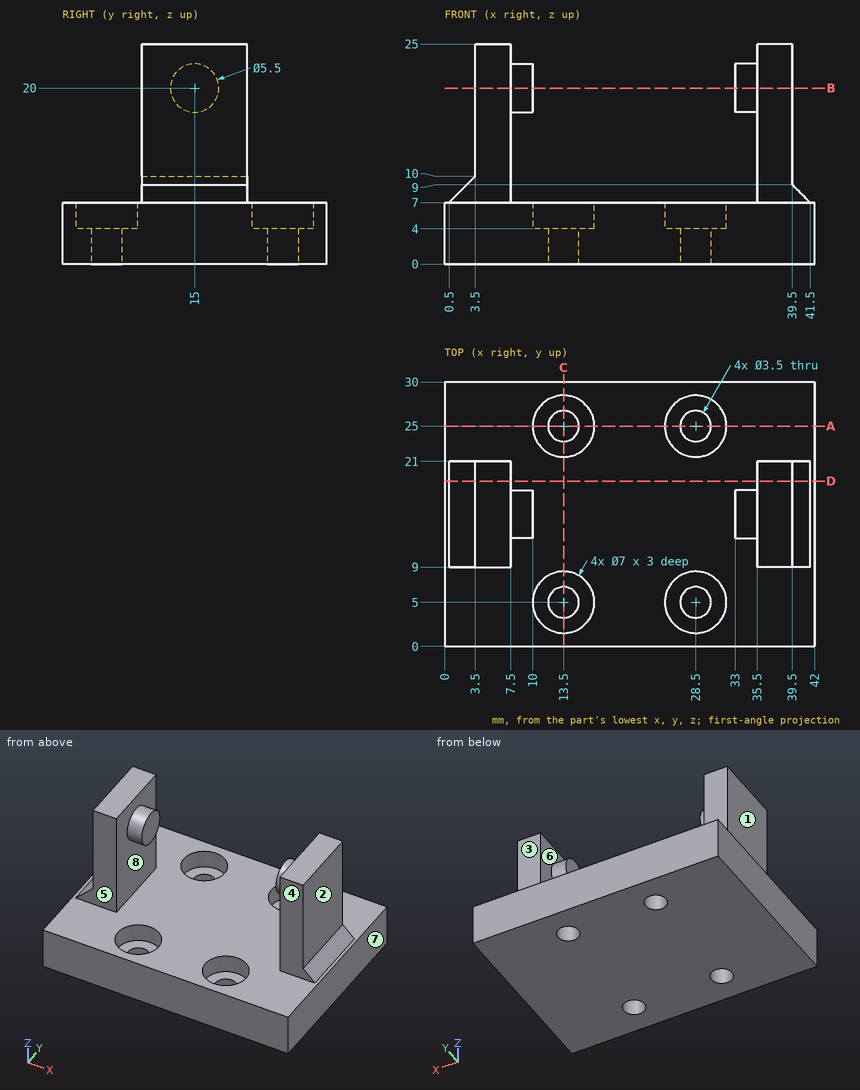
Design review of the part shown in the three views and the two pictorial views. Dimensions are in mm from the part's minimum x, y and z. A direction names the side the tool comes from. Round coordinates to 2 decimals unless told otherwise and drop trailing zeros. Write each loop counter-clockwise with the first axis right and the second up, starting at its lowest first coordinate (ties: lowest second). Pieces come first, ordered by that corner, then holes. Notation, with made-up numbers: M 73.25,42.5 L 118.25,42.5 A26 ccw 118.25,79.5 Z; hole C 33,46 d2. An arc over 180 degrees is marked long. One line per item, written item: value. Start each with the question number.
1. Take a section at B-B on z = 20. State the section outline as (x, y) points, then the cut area to 4 significant figures.
2. Take a section at D-D on y = 18.75. State the section outline as (x, z) points.
3. To check wall thickness, follow probe 1 along Y at (x, z) = (28.5, 0.9); probe 2 along Y at (x, z) = (12, 3.75); probe 3 along X at (y, z) = (19.25, 22). State the ranges of each line that lie inside material, in increasing order. Write a range as from..to.
4. Take a section at C-C on x = 13.5. State the section outline as (y, z) points.
5. Draft analysis for pull direction X (two halves, no side actions). For the marked faces 5, 6, 7 and 8, state which applies: pulls with the +X half, pulls with the -X half, needs draft (parallel to the pull), parting line crosses it, or undercut.
6. Clearance check with flat-ended pins moving along their axes: P1, Ø3, axis at x = 35, y = 24.5, coming from the +Z side; P2, Ø2, axis at x = 5, z = 11.5, coming from the +Y side; P3, Ø5.5, axis at x = 5, z = 18.5, coming from the -Y side; P4, Ø2, axis at x = 13.5, y = 5, coming from the -Z side. State where each tip first meets the part, or that it passes through.
7. Take a section at A-A on y = 25. State the section outline as (x, z) points, then the cut area to 3 significant figures.
8. For the marked faces 1, 2, 3 and 4, list the 3-axis set-ups (+Z, -Z, +X, -X, +Y, -Y) from which the entire face can be reached by the end or side of a thin tool; tool diameter is ignored.
Computed:
1. outline: M 3.5,9 L 7.5,9 L 7.5,12.25 L 10,12.25 L 10,17.75 L 7.5,17.75 L 7.5,21 L 3.5,21 Z; M 33,12.25 L 35.5,12.25 L 35.5,9 L 39.5,9 L 39.5,21 L 35.5,21 L 35.5,17.75 L 33,17.75 Z
1. area: 123.5 mm²
2. outline: M 0,0 L 42,0 L 42,7 L 41.5,7 L 39.5,9 L 39.5,25 L 35.5,25 L 35.5,7 L 7.5,7 L 7.5,25 L 3.5,25 L 3.5,10 L 0.5,7 L 0,7 Z
3. probe 1: y = 0..3.25, 6.75..23.25, 26.75..30
3. probe 2: y = 0..4.1, 5.9..24.1, 25.9..30
3. probe 3: x = 3.5..7.5, 35.5..39.5
4. outline: M 0,0 L 3.25,0 L 3.25,4 L 1.5,4 L 1.5,7 L 0,7 Z; M 6.75,0 L 23.25,0 L 23.25,4 L 21.5,4 L 21.5,7 L 8.5,7 L 8.5,4 L 6.75,4 Z; M 26.75,0 L 30,0 L 30,7 L 28.5,7 L 28.5,4 L 26.75,4 Z
5. face 5: needs draft
5. face 6: undercut
5. face 7: pulls with the +X half
5. face 8: undercut
6. P1: stops at z = 7
6. P2: stops at y = 21
6. P3: stops at y = 9
6. P4: passes through
7. outline: M 0,0 L 11.75,0 L 11.75,4 L 10,4 L 10,7 L 0,7 Z; M 15.25,0 L 26.75,0 L 26.75,4 L 25,4 L 25,7 L 17,7 L 17,4 L 15.25,4 Z; M 30.25,0 L 42,0 L 42,7 L 32,7 L 32,4 L 30.25,4 Z
7. area: 224 mm²
8. face 1: +Z, -X, +Y, -Y
8. face 2: +Z, +X, +Y, -Y
8. face 3: +Z, +X, -X, +Y
8. face 4: +Z, +X, -X, -Y
